Job drawing, mm, ordinate dimensions from the low corner. One solid piece. A direction names the side the tool comes from. Give positions to 0.01 mm unless a question says otherwise; leave off trailing zeros. Write each loop counter-clockwise with the first axis right and the second up, starting at its lowest first coordinate (ties: lowest second). Pieces come first, ordered by that corner, then holes. Notation, with made-up numbers: M 73,18.5 L 90,18.5 A36 cw 90,53.5 Z; hole C 72,-21.5 d3. An arc over 180 degrees is marked long. Answer as CSV lines item,"result". Start each with the question number.
Item 1: Band-saw the part on C-C, the plane x = 114. List the corners of the cut face in (y, z).
Item 2: Band-saw the part on D-D, the plane y = 34. List the corners of the cut face in (x, z), then the cut area to 3 significant figures.
Item 3: Pin check, flat tips, straight feed: pin 1 (4 mm diameter, centred on x = 92, y = 55, fed in from -Z); pin 2 (2 mm diameter, centred on x = 86, z = 177, fed in from +Y). Stop position of each tip, or through.
Item 4: Band-saw the part on B-B, the plane z = 158. List the corners of the cut face in (x, y), then the cut area to 3 significant figures.
Item 5: 3-axis set-ups, long thin cutter, end or side, ignore diameter. For the marked faces 1, 2 and 3: which of +Z, -Z, +X, -X, +Y, -Y reach the whole face in a straight line?
Item 6: Wall check: L1, parallel to X at y = 64.5, z = 141.5; L2, parallel to X at y = 60.5, z = 22.5 (1 decimal); L3, parallel to Z at x = 158.5, y = 69. Give the ranges that are in metal, low to high. Write a range as from..to.
Item 7: Band-saw the part on A-A, the plane y = 60. List the corners of the cut face in (x, z) (1 decimal).
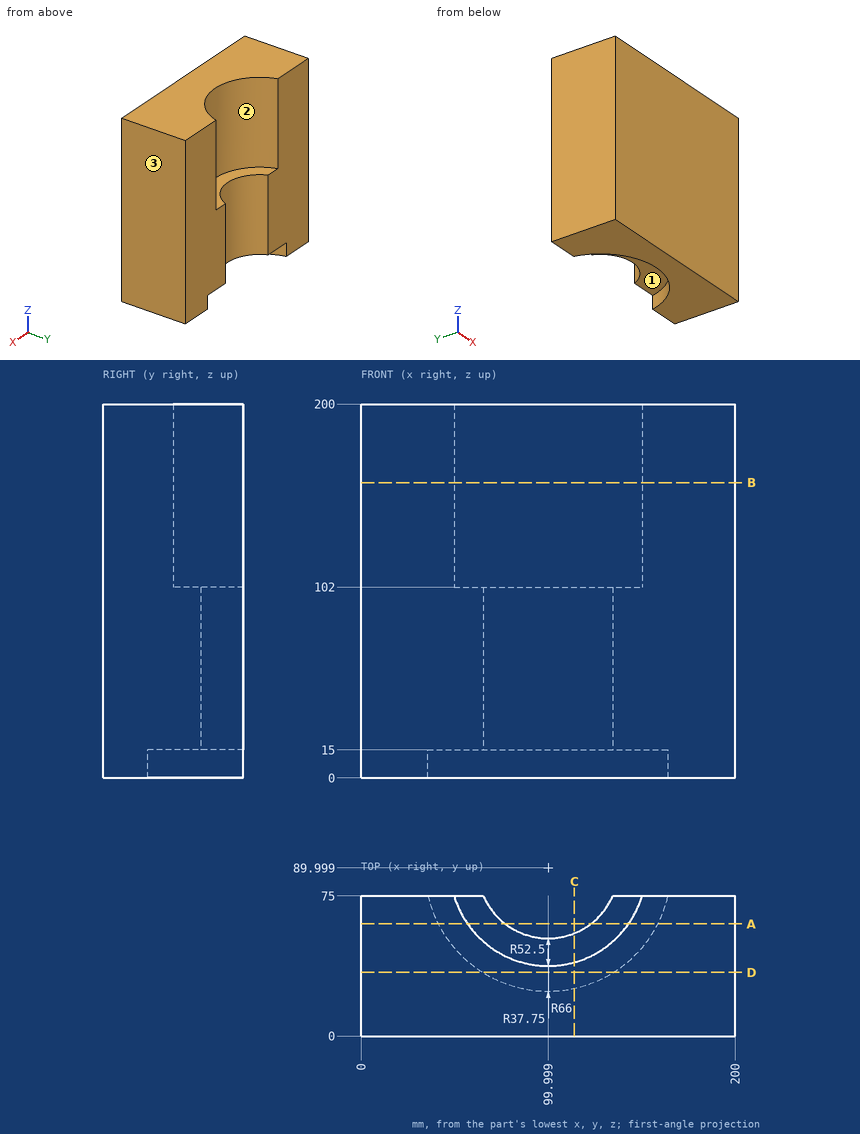
Output:
1,outline,"M 0,0 L 25.5,0 L 25.5,15 L 54.94,15 L 54.94,102 L 39.4,102 L 39.4,200 L 0,200 Z"
2,outline,"M 0,0 L 65.07,0 L 65.07,15 L 134.93,15 L 134.93,0 L 200,0 L 200,200 L 0,200 Z"
2,area,"39,000 mm²"
3,pin 1,"z = 15"
3,pin 2,"y = 39.69"
4,outline,"M 0,0 L 200,0 L 200,75 L 150.31,75 A52.5 cw 49.69,75 L 0,75 Z"
4,area,"12,200 mm²"
5,face 1,"-Z, +Y"
5,face 2,"+Z, +Y"
5,face 3,"+Z, -Z, +X, +Y, -Y"
6,L1,"0..54.11, 145.89..200"
6,L2,"0..76.4, 123.6..200"
6,L3,"15..200"
7,outline,"M 0,0 L 41.2,0 L 41.2,15 L 77.1,15 L 77.1,102 L 56.9,102 L 56.9,200 L 0,200 Z; M 122.9,15 L 158.8,15 L 158.8,0 L 200,0 L 200,200 L 143.1,200 L 143.1,102 L 122.9,102 Z"
